Geometry check sheet. Reference: drawing and pictorial views, mm from the part's lowest x, y, z. A direction names the side the tool comes from. Give positions to 0.01 mm unless a question says otherwise; leave off trailing zeros. Loops run counter-clockwise (first coordinate to the right, second up) from the corner with the lowest first, then second, coordinate; pieces in that order, holes last. Notation, with made-up numbers: M 76.25,7.25 L 121.25,7.25 A16 ccw 121.25,22.25 Z; hole C 64,57.25 d7. An arc over 180 degrees is marked long. Put each result on its own line as item: value. Start each with the question number.
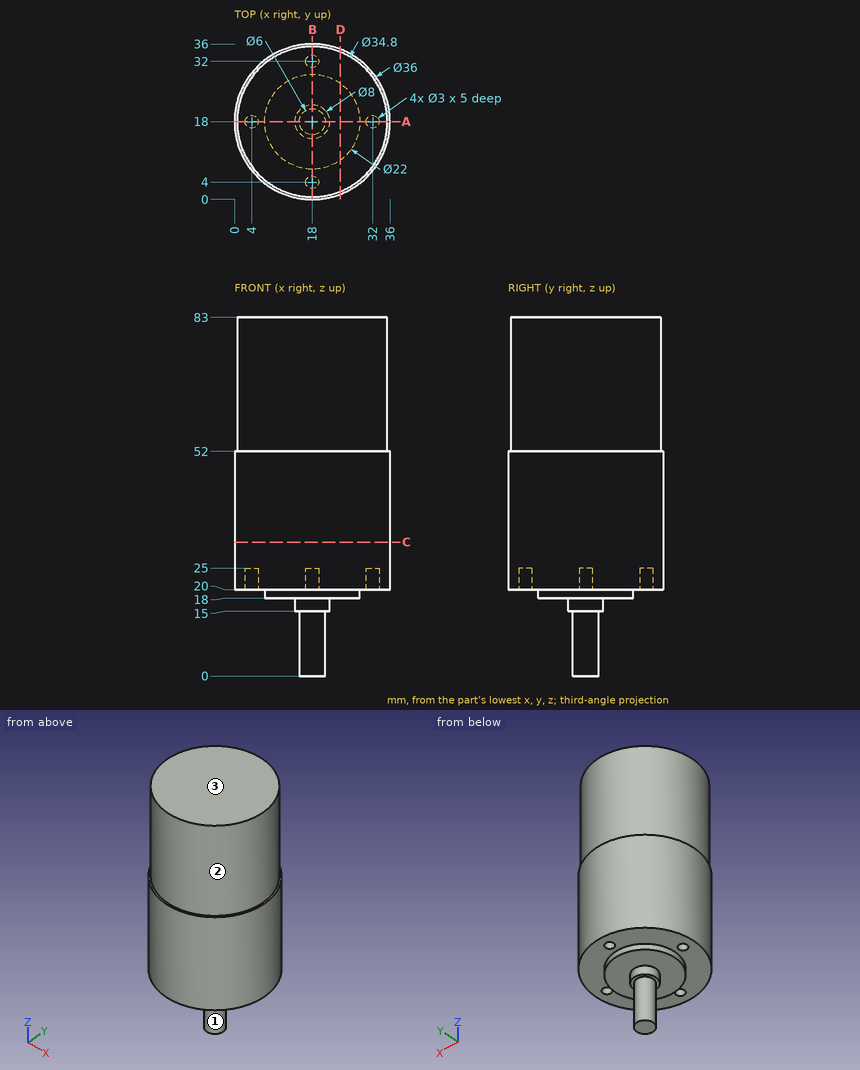
Q1. Thickness scan on line 1 along Y through (x, z) = (18, 23); line 2 along Z through (x, y) = (9, 5); line 3 along Z through (x, y) = (5, 17.5). Record the ranges inside material, lowest first. Write a range as [from, to].
Q2. Section check A-A, the plane y = 18. Record the cut outline in (x, z).
Q3. Section check D-D, the plane x = 24.5. Record the cut outline in (y, z), then the cut area to 3 significant figures.
Q4. Depth check by flat-ended pin: P1, Ø5, axis at x = 4, y = 18, coming from the -Z side; P2, Ø4, axis at x = 22.5, z = 39, coming from the -Y side; P3, Ø5, axis at x = 28.5, y = 25, coming from the -Z side. Enter the tip coordinate at first touch or a pass-through.
Q5. Access from +Z, -Z, +X, -X, +Y, -Y to the whole of each face (thin tool, end or side, straight path). Record for the marked faces 1, 2 and 3.
Q6. Section check C-C, the plane z = 31. Record the cut outline in (x, y).
Found:
1. line 1: y = [0, 2.5], [5.5, 30.5], [33.5, 36]
1. line 2: z = [20, 83]
1. line 3: z = [25, 83]
2. outline: M 0,20 L 2.5,20 L 2.5,25 L 5.5,25 L 5.5,20 L 7,20 L 7,18 L 14,18 L 14,15 L 15,15 L 15,0 L 21,0 L 21,15 L 22,15 L 22,18 L 29,18 L 29,20 L 30.5,20 L 30.5,25 L 33.5,25 L 33.5,20 L 36,20 L 36,52 L 35.4,52 L 35.4,83 L 0.6,83 L 0.6,52 L 0,52 Z
3. outline: M 1.21,20 L 9.13,20 L 9.13,18 L 26.87,18 L 26.87,20 L 34.79,20 L 34.79,52 L 34.14,52 L 34.14,83 L 1.86,83 L 1.86,52 L 1.21,52 Z
3. area: 2,110 mm^2
4. P1: stops at z = 20
4. P2: stops at y = 0.17
4. P3: stops at z = 18
5. face 1: -Z
5. face 2: +Z
5. face 3: +Z, +X, -X, +Y, -Y
6. outline: C 18,18 d36
